Autodesk Inventor part; units mm, degrees
ref_plane "YZ Plane" through (0, 0, 0) normal (1, 0, 0) x (0, 1, 0)
ref_plane "XZ Plane" through (0, 0, 0) normal (0, 1, 0) x (-1, 0, 0)
ref_plane "XY Plane" through (0, 0, 0) normal (0, 0, 1) x (1, 0, 0)
sketch "Sketch2" plane through (0, 0, 0) normal (0, 0, 1) x (1, 0, 0)
  line L0 (0, 0) -> (0, 25.4)
  line L1 (0, 25.4) -> (7.62, 25.4)
  line L2 (7.62, 25.4) -> (9.144, 25.4)
  line L3 (10.9873, 24.8102) -> (46.2933, -0.3635)
  line L4 (40.6545, 1.846) -> (7.62, 25.4)
  line L5 (47.625, -2.9486) -> (47.625, -12.4656)
  line L6 (10.9873, 24.8102) -> (11.4917, 24.4504)
  line L7 (9.144, 25.4) -> (10.16, 25.4)
  line L8 (10.16, 27.0356) -> (10.16, 47.625)
  line L9 (7.62, 50.8) -> (7.62, 25.4)
  line L10 (45.9232, -2.5626) -> (45.9232, -11.4526)
  arc A0 (10.16, 47.625) -> (7.62, 50.7359) centre (6.985, 47.625) ccw
  arc A1 (47.625, -2.9486) -> (46.2933, -0.3635) centre (44.45, -2.9486) ccw
  arc A2 (10.16, 27.0356) -> (11.4917, 24.4504) centre (13.335, 27.0356) ccw
  line L11 (40.6545, 1.846) -> (45.9232, -2.5626)
  line L12 (47.625, -12.4656) -> (45.9232, -11.4526)
  line L13 (45.9232, -2.5626) -> (45.9232, -11.4526)
  line L14 (45.5168, -35.3256) -> (45.5168, -16.9106)
  line L15 (47.625, -12.4656) -> (52.4025, -12.4656) construction
  line L16 (43.8086, -35.3256) -> (43.8086, -15.9112)
  line L17 (45.9232, -2.5626) -> (45.9232, -11.4526)
  line L18 (45.5168, -35.3256) -> (43.8086, -35.3256)
  line L19 (45.5168, -16.9106) -> (45.5168, -35.3256)
  line L20 (47.625, -12.4656) -> (45.5168, -16.9106)
  line L21 (45.9232, -11.4526) -> (43.8086, -15.9112)
  line L22 (7.62, 25.4) -> (3.81, 25.4)
  line L23 (3.81, 25.4) -> (3.81, 32.3365)
  line L24 (7.62, 25.4) -> (3.81, 28.1166)
  line L25 (3.81, 28.1166) -> (7.62, 28.1166)
  point P0 (47.625, -1.313)
  point P1 (10.16, 50.8)
  point P2 (46.1518, -17.3808)
  point P3 (44.9154, -1.7193)
  point P4 (46.1518, -15.158)
  point P5 (42.6103, 0.2095)
  dimension "d9" = 25.4
  dimension "d10" = 7.62
  dimension "d11" = 2.54
  dimension "d16" = 25.4
  dimension "d18" = 3.175
  dimension "d19" = 3.175
  dimension "d24" = 47.625
  dimension "d26" = 8.89
  dimension "d53" = 45.5168
  dimension "d55" = 1.7082
  dimension "d56" = 22.86
  dimension "d68" = 1.7018
  dimension "d84" = 18.415
  dimension "d86" = 3.81
ref_plane "Work Plane1" through (0, -36.5956, 0) normal (0, -1, 0) x (1, 0, 0)
revolve "Revolution5" add sketch "Sketch2" angle 360 about axis through (0, 0, 0) along (0, 1, 0) contours L9 A0 L8 A2 L3 A1 L5 L12 L10 L11 L4 | L24 L25 L9 | L12 L20 L14 L18 L16 L21
sketch "Sketch8" plane through (0, -35.3256, 0) normal (0, -1, 0) x (1, 0, 0)
  circle A0 centre (0, 0) radius 43.8086
  line L0 (0, 43.8086) -> (0, 46.5836)
  line L1 (41.6644, 13.5376) -> (44.3484, 14.2568)
  line L2 (43.8086, 0) -> (46.5836, 0) construction
  line L3 (0, 0) -> (46.5836, 0)
  line L4 (-13.6758, 41.6193) -> (-14.3951, 44.3036)
  line L5 (0, 0) -> (46.5836, 0) construction
  line L6 (-43.8086, 0) -> (-46.5836, 0)
  line L7 (-41.6193, -13.6758) -> (-44.3036, -14.3951)
  line L8 (0, 0) -> (46.5836, 0) construction
  line L9 (0, -43.8086) -> (0, -46.5836)
  line L10 (13.5376, -41.6644) -> (14.2568, -44.3484)
  line L11 (0, 0) -> (46.5836, 0) construction
  arc A1 (0, 46.5836) -> (-14.3951, 44.3036) centre (0, 0) ccw
  arc A2 (-46.5836, 0) -> (-44.3036, -14.3951) centre (0, 0) ccw
  arc A3 (0, -46.5836) -> (14.2568, -44.3484) centre (0, 0) ccw
  arc A4 (46.5836, 0) -> (44.3484, 14.2568) centre (0, 0) ccw
  arc A5 (0, -43.8086) -> (13.5376, -41.6644) centre (0, 0) ccw
  arc A6 (-43.8086, 0) -> (-41.6193, -13.6758) centre (0, 0) ccw
  arc A7 (43.8086, 0) -> (41.6644, 13.5376) centre (0, 0) ccw
  arc A8 (0, 43.8086) -> (-13.6758, 41.6193) centre (0, 0) ccw
  line L12 (46.5836, 0) -> (43.8086, 0)
  circle A9 centre (0, 0) radius 45.5168
  circle A10 centre (0, 0) radius 41.275
  dimension "d72" = 15
  dimension "d75" = 105
  dimension "d78" = 165
  dimension "d81" = 75
  dimension "d85" = 82.55
extrude "Extrusion7" add sketch "Sketch8" against normal blind 2.54 contours A0 | A0 L1 A9 L3 | L10 A9 L9 A0 | A9 L1 A4 L3 | A0 L4 A9 L0 | L10 A3 L9 A9 | A9 L4 A1 L0 | L7 A9 L6 A0 | L7 A2 L6 A9
properties part number "screwflare74"
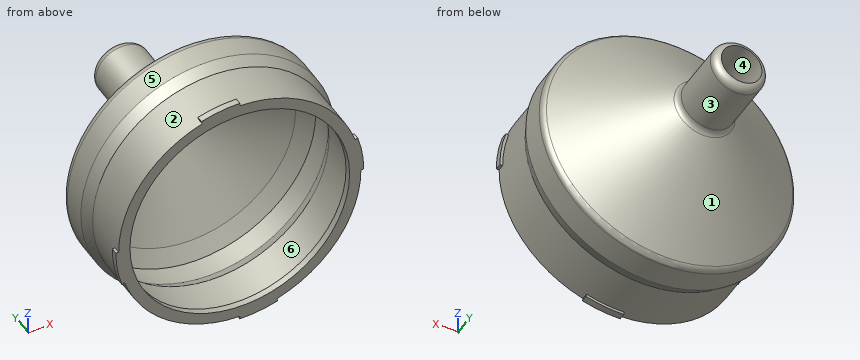
Could you check a few things on this model? Use its own coordinates, in mm. Face numbers are marked on the shaded views. A direction names the side the tool comes from. Give positions to 0.01 mm unless a question says otherwise; leave off trailing zeros. Order: outer loops, then holes, each group sorted by start corner. A loop starts at its lowest first (then second) coordinate and runs counter-clockwise, first axis right, second up.
1. Suppose I cut it at A-A (y = 41). Write out the boundary of the cut face in (x, z).
Answers below:
outline: circle Ø20.32 at (0, 0); hole circle Ø15.24 at (0, 0)
2. For pin 1 (12 mm diameter, centred on x = 0.5, z = -3, fed in from +Y); pin 2 (3 mm diameter, centred on y = -14, z = 27, fed in from +X); pin 3 (1.5 mm diameter, centred on x = -4.5, y = 28, fed in from +Z); pin 4 (2.5 mm diameter, centred on x = -45.5, z = -5.5, fed in from +Y), each with a flat end and sliding along its axis, tell me the tip position at first contact or that it passes through.
Answers below:
pin 1: stops at y = 50.74
pin 2: stops at x = 39.68
pin 3: stops at z = 9.44
pin 4: stops at y = 0.86
3. I need wall thicknesses on L1, parallel to X at y = 44, z = 0; L2, parallel to Z at x = 0, y = -7.25 (3 decimals). Which ranges of each line are inside material? Lowest first, please.
Answers below:
L1: x = -10.16 to -7.62, 7.62 to 10.16
L2: z = -47.625 to -45.923, 45.923 to 47.625
4. Which directions (+Z, -Z, +X, -X, +Y, -Y) give clear straight access to the entire face, cutting with the end or side of a thin tool? Please do the marked faces 4, 5 and 6.
Answers below:
face 4: +Y
face 5: +Y, -Y
face 6: none
5. Thinking about a two-plate mould opening in Y: for the marked faces 1, 2 and 3, which applies, +Y half, -Y half, draft (parallel to the pull), parting line (faces both ways), or undercut?
Answers below:
face 1: +Y half
face 2: undercut
face 3: draft
6. Suppose I cut it at B-B (y = 15). Write out the boundary of the cut face in (x, z).
Answers below:
outline: circle Ø49.49 at (0, 0); hole circle Ø44.41 at (0, 0)
